```python
from build123d import *

# Parameters (mm, degrees)
SKETCH1_W                     = 965
SKETCH1_H                     = 279
BASE_FLANGE1_DEPTH            = 0.7366
EDGE_FLANGE1_STRIP_W          = 4.4196
EDGE_FLANGE1_STRIP_H          = 0.7366
EDGE_FLANGE1_STRIP_CUT_DEPTH  = 965
EDGE_FLANGE1_DEPTH            = 965
EDGE_FLANGE2_STRIP_W          = 4.4196
EDGE_FLANGE2_STRIP_H          = 0.7366
EDGE_FLANGE2_STRIP_CUT_DEPTH  = 277.5268
EDGE_FLANGE2_DEPTH            = 277.5268
EDGE_FLANGE3_STRIP_W          = 4.4196
EDGE_FLANGE3_STRIP_H          = 0.7366
EDGE_FLANGE3_STRIP_CUT_DEPTH  = 963.5268
EDGE_FLANGE3_DEPTH            = 963.5268
EDGE_FLANGE4_STRIP_W          = 4.4196
EDGE_FLANGE4_STRIP_H          = 0.7366
EDGE_FLANGE4_STRIP_CUT_DEPTH  = 276.0536
EDGE_FLANGE4_DEPTH            = 276.0536
EDGE_FLANGE5_STRIP_W          = 4.4196
EDGE_FLANGE5_STRIP_H          = 0.7366
EDGE_FLANGE5_STRIP_CUT_DEPTH  = 903.1268
EDGE_FLANGE5_RELIEF_W         = 4.7879
EDGE_FLANGE5_RELIEF_H         = 0.3683
EDGE_FLANGE5_RELIEF_CUT_DEPTH = 0.7366
EDGE_FLANGE5_DEPTH            = 903.1268
EDGE_FLANGE6_STRIP_W          = 4.4196
EDGE_FLANGE6_STRIP_H          = 0.7366
EDGE_FLANGE6_STRIP_CUT_DEPTH  = 903.1268
EDGE_FLANGE6_RELIEF_W         = 4.7879
EDGE_FLANGE6_RELIEF_H         = 0.3683
EDGE_FLANGE6_RELIEF_CUT_DEPTH = 0.7366
EDGE_FLANGE6_DEPTH            = 903.1268
EDGE_FLANGE7_STRIP_W          = 4.4196
EDGE_FLANGE7_STRIP_H          = 0.7366
EDGE_FLANGE7_STRIP_CUT_DEPTH  = 276.5902
EDGE_FLANGE7_RELIEF_W         = 4.7879
EDGE_FLANGE7_RELIEF_H         = 0.3683
EDGE_FLANGE7_RELIEF_CUT_DEPTH = 0.7366
EDGE_FLANGE7_DEPTH            = 276.5902
EDGE_FLANGE7_PROFILE_W        = 276.6268
EDGE_FLANGE7_PROFILE_H        = 28.5268
EDGE_FLANGE7_FLAT_DEPTH       = 0.7366
EDGE_FLANGE8_STRIP_W          = 4.4196
EDGE_FLANGE8_STRIP_H          = 0.7366
EDGE_FLANGE8_STRIP_CUT_DEPTH  = 276.0536
EDGE_FLANGE8_DEPTH            = 276.0536


# Sheet-metal steps are written as plain solids
with BuildPart() as part:
    # Sketch1 → Base-Flange1 (new body)
    with BuildSketch(Plane.XY):
        Rectangle(SKETCH1_W, SKETCH1_H)
    extrude(amount=-BASE_FLANGE1_DEPTH)

    # Edge-Flange1 strip (across the edge) → Edge-Flange1 strip cut (cut)
    with BuildSketch(Plane(origin=(-482.5, 139.5, -0.7366), x_dir=(0, -1, 0), z_dir=(1, 0, 0))):
        with Locations((-0.7366, -0.3683)):
            Rectangle(EDGE_FLANGE1_STRIP_W, EDGE_FLANGE1_STRIP_H)
    extrude(amount=EDGE_FLANGE1_STRIP_CUT_DEPTH, mode=Mode.SUBTRACT)

    # Edge-Flange1 section (across the edge) → Edge-Flange1 (add)
    with BuildSketch(Plane(origin=(-482.5, 139.5, -0.7366), x_dir=(0, -1, 0), z_dir=(1, 0, 0))):
        with BuildLine():
            Line((0, 0.7366), (0, 29.2634))
            Line((0, 29.2634), (0.7366, 29.2634))
            Line((0.7366, 29.2634), (0.7366, 0.7366))
            ThreePointArc((0.7366, 0.7366), (0.952345145, 0.215745145), (1.4732, 0))
            Line((1.4732, 0), (1.4732, -0.7366))
            ThreePointArc((1.4732, -0.7366), (0.43149029, -0.30510971), (0, 0.7366))
        make_face()
    extrude(amount=EDGE_FLANGE1_DEPTH)

    # Edge-Flange2 strip (across the edge) → Edge-Flange2 strip cut (cut)
    with BuildSketch(Plane(origin=(482.5, 138.0268, -0.7366), x_dir=(-1, 0, 0), z_dir=(0, -1, 0))):
        with Locations((-0.7366, -0.3683)):
            Rectangle(EDGE_FLANGE2_STRIP_W, EDGE_FLANGE2_STRIP_H)
    extrude(amount=EDGE_FLANGE2_STRIP_CUT_DEPTH, mode=Mode.SUBTRACT)

    # Edge-Flange2 section (across the edge) → Edge-Flange2 (add)
    with BuildSketch(Plane(origin=(482.5, 138.0268, -0.7366), x_dir=(-1, 0, 0), z_dir=(0, -1, 0))):
        with BuildLine():
            Line((0, 0.7366), (0, 29.2634))
            Line((0, 29.2634), (0.7366, 29.2634))
            Line((0.7366, 29.2634), (0.7366, 0.7366))
            ThreePointArc((0.7366, 0.7366), (0.952345145, 0.215745145), (1.4732, 0))
            Line((1.4732, 0), (1.4732, -0.7366))
            ThreePointArc((1.4732, -0.7366), (0.43149029, -0.30510971), (0, 0.7366))
        make_face()
    extrude(amount=EDGE_FLANGE2_DEPTH)

    # Edge-Flange3 strip (across the edge) → Edge-Flange3 strip cut (cut)
    with BuildSketch(Plane(origin=(481.0268, -139.5, -0.7366), x_dir=(0, 1, 0), z_dir=(-1, 0, 0))):
        with Locations((-0.7366, -0.3683)):
            Rectangle(EDGE_FLANGE3_STRIP_W, EDGE_FLANGE3_STRIP_H)
    extrude(amount=EDGE_FLANGE3_STRIP_CUT_DEPTH, mode=Mode.SUBTRACT)

    # Edge-Flange3 section (across the edge) → Edge-Flange3 (add)
    with BuildSketch(Plane(origin=(481.0268, -139.5, -0.7366), x_dir=(0, 1, 0), z_dir=(-1, 0, 0))):
        with BuildLine():
            Line((0, 0.7366), (0, 29.2634))
            Line((0, 29.2634), (0.7366, 29.2634))
            Line((0.7366, 29.2634), (0.7366, 0.7366))
            ThreePointArc((0.7366, 0.7366), (0.952345145, 0.215745145), (1.4732, 0))
            Line((1.4732, 0), (1.4732, -0.7366))
            ThreePointArc((1.4732, -0.7366), (0.43149029, -0.30510971), (0, 0.7366))
        make_face()
    extrude(amount=EDGE_FLANGE3_DEPTH)

    # Edge-Flange4 strip (across the edge) → Edge-Flange4 strip cut (cut)
    with BuildSketch(Plane(origin=(-482.5, -138.0268, -0.7366), x_dir=(1, 0, 0), z_dir=(0, 1, 0))):
        with Locations((-0.7366, -0.3683)):
            Rectangle(EDGE_FLANGE4_STRIP_W, EDGE_FLANGE4_STRIP_H)
    extrude(amount=EDGE_FLANGE4_STRIP_CUT_DEPTH, mode=Mode.SUBTRACT)

    # Edge-Flange4 section (across the edge) → Edge-Flange4 (add)
    with BuildSketch(Plane(origin=(-482.5, -138.0268, -0.7366), x_dir=(1, 0, 0), z_dir=(0, 1, 0))):
        with BuildLine():
            Line((0, 0.7366), (0, 29.2634))
            Line((0, 29.2634), (0.7366, 29.2634))
            Line((0.7366, 29.2634), (0.7366, 0.7366))
            ThreePointArc((0.7366, 0.7366), (0.952345145, 0.215745145), (1.4732, 0))
            Line((1.4732, 0), (1.4732, -0.7366))
            ThreePointArc((1.4732, -0.7366), (0.43149029, -0.30510971), (0, 0.7366))
        make_face()
    extrude(amount=EDGE_FLANGE4_DEPTH)

    # Edge-Flange5 strip (across the edge) → Edge-Flange5 strip cut (cut)
    with BuildSketch(Plane(origin=(451.5634, -138.7634, -30), x_dir=(0, 0, 1), z_dir=(-1, 0, 0))):
        with Locations((-0.7366, -0.3683)):
            Rectangle(EDGE_FLANGE5_STRIP_W, EDGE_FLANGE5_STRIP_H)
    extrude(amount=EDGE_FLANGE5_STRIP_CUT_DEPTH, mode=Mode.SUBTRACT)

    # Edge-Flange5 relief (on the sheet) → Edge-Flange5 relief cut (cut)
    with BuildSketch(Plane(origin=(451.5634, -138.7634, -28.5268), x_dir=(0, 0, 1), z_dir=(0, 1, 0))):
        with Locations((-2.02565, 0.18415)):
            Rectangle(EDGE_FLANGE5_RELIEF_W, EDGE_FLANGE5_RELIEF_H)
        with Locations((-2.02565, -903.31095)):
            Rectangle(EDGE_FLANGE5_RELIEF_W, EDGE_FLANGE5_RELIEF_H)
    extrude(amount=-EDGE_FLANGE5_RELIEF_CUT_DEPTH, mode=Mode.SUBTRACT)

    # Edge-Flange5 section (across the edge) → Edge-Flange5 (add)
    with BuildSketch(Plane(origin=(451.5634, -138.7634, -30), x_dir=(0, 0, 1), z_dir=(-1, 0, 0))):
        with BuildLine():
            Line((0, 0.7366), (0, 29.2634))
            Line((0, 29.2634), (0.7366, 29.2634))
            Line((0.7366, 29.2634), (0.7366, 0.7366))
            ThreePointArc((0.7366, 0.7366), (0.952345145, 0.215745145), (1.4732, 0))
            Line((1.4732, 0), (1.4732, -0.7366))
            ThreePointArc((1.4732, -0.7366), (0.43149029, -0.30510971), (0, 0.7366))
        make_face()
    extrude(amount=EDGE_FLANGE5_DEPTH)

    # Edge-Flange6 strip (across the edge) → Edge-Flange6 strip cut (cut)
    with BuildSketch(Plane(origin=(-451.5634, 138.7634, -30), x_dir=(0, 0, 1), z_dir=(1, 0, 0))):
        with Locations((-0.7366, -0.3683)):
            Rectangle(EDGE_FLANGE6_STRIP_W, EDGE_FLANGE6_STRIP_H)
    extrude(amount=EDGE_FLANGE6_STRIP_CUT_DEPTH, mode=Mode.SUBTRACT)

    # Edge-Flange6 relief (on the sheet) → Edge-Flange6 relief cut (cut)
    with BuildSketch(Plane(origin=(-451.5634, 138.7634, -28.5268), x_dir=(0, 0, 1), z_dir=(0, -1, 0))):
        with Locations((-2.02565, 0.18415)):
            Rectangle(EDGE_FLANGE6_RELIEF_W, EDGE_FLANGE6_RELIEF_H)
        with Locations((-2.02565, -903.31095)):
            Rectangle(EDGE_FLANGE6_RELIEF_W, EDGE_FLANGE6_RELIEF_H)
    extrude(amount=-EDGE_FLANGE6_RELIEF_CUT_DEPTH, mode=Mode.SUBTRACT)

    # Edge-Flange6 section (across the edge) → Edge-Flange6 (add)
    with BuildSketch(Plane(origin=(-451.5634, 138.7634, -30), x_dir=(0, 0, 1), z_dir=(1, 0, 0))):
        with BuildLine():
            Line((0, 0.7366), (0, 29.2634))
            Line((0, 29.2634), (0.7366, 29.2634))
            Line((0.7366, 29.2634), (0.7366, 0.7366))
            ThreePointArc((0.7366, 0.7366), (0.952345145, 0.215745145), (1.4732, 0))
            Line((1.4732, 0), (1.4732, -0.7366))
            ThreePointArc((1.4732, -0.7366), (0.43149029, -0.30510971), (0, 0.7366))
        make_face()
    extrude(amount=EDGE_FLANGE6_DEPTH)

    # Edge-Flange7 strip (across the edge) → Edge-Flange7 strip cut (cut)
    with BuildSketch(Plane(origin=(481.7634, 138.0268, -30), x_dir=(0, 0, 1), z_dir=(0, -1, 0))):
        with Locations((-0.7366, -0.3683)):
            Rectangle(EDGE_FLANGE7_STRIP_W, EDGE_FLANGE7_STRIP_H)
    extrude(amount=EDGE_FLANGE7_STRIP_CUT_DEPTH, mode=Mode.SUBTRACT)

    # Edge-Flange7 relief (on the sheet) → Edge-Flange7 relief cut (cut)
    with BuildSketch(Plane(origin=(481.7634, 138.0268, -28.5268), x_dir=(0, 0, 1), z_dir=(-1, 0, 0))):
        with Locations((-2.02565, -276.77435)):
            Rectangle(EDGE_FLANGE7_RELIEF_W, EDGE_FLANGE7_RELIEF_H)
    extrude(amount=-EDGE_FLANGE7_RELIEF_CUT_DEPTH, mode=Mode.SUBTRACT)

    # Edge-Flange7 bend section (across the edge) → Edge-Flange7 (add)
    with BuildSketch(Plane(origin=(481.7634, 138.0268, -30), x_dir=(0, 0, 1), z_dir=(0, -1, 0))):
        with BuildLine():
            Line((0, 0.7366), (0.7366, 0.7366))
            ThreePointArc((0.7366, 0.7366), (0.952345145, 0.215745145), (1.4732, 0))
            Line((1.4732, 0), (1.4732, -0.7366))
            ThreePointArc((1.4732, -0.7366), (0.43149029, -0.30510971), (0, 0.7366))
        make_face()
    extrude(amount=EDGE_FLANGE7_DEPTH)

    # Edge-Flange7 profile (on flange) → Edge-Flange7 flat (add)
    with BuildSketch(Plane(origin=(481.7634, 0, -30), x_dir=(0, 1, 0), z_dir=(0, 0, 1))):
        with Locations((-0.25, 15)):
            Rectangle(EDGE_FLANGE7_PROFILE_W, EDGE_FLANGE7_PROFILE_H)
    extrude(amount=EDGE_FLANGE7_FLAT_DEPTH)

    # Edge-Flange8 strip (across the edge) → Edge-Flange8 strip cut (cut)
    with BuildSketch(Plane(origin=(-481.7634, -138.0268, -30), x_dir=(0, 0, 1), z_dir=(0, 1, 0))):
        with Locations((-0.7366, -0.3683)):
            Rectangle(EDGE_FLANGE8_STRIP_W, EDGE_FLANGE8_STRIP_H)
    extrude(amount=EDGE_FLANGE8_STRIP_CUT_DEPTH, mode=Mode.SUBTRACT)

    # Edge-Flange8 section (across the edge) → Edge-Flange8 (add)
    with BuildSketch(Plane(origin=(-481.7634, -138.0268, -30), x_dir=(0, 0, 1), z_dir=(0, 1, 0))):
        with BuildLine():
            Line((0, 0.7366), (0, 29.2634))
            Line((0, 29.2634), (0.7366, 29.2634))
            Line((0.7366, 29.2634), (0.7366, 0.7366))
            ThreePointArc((0.7366, 0.7366), (0.952345145, 0.215745145), (1.4732, 0))
            Line((1.4732, 0), (1.4732, -0.7366))
            ThreePointArc((1.4732, -0.7366), (0.43149029, -0.30510971), (0, 0.7366))
        make_face()
    extrude(amount=EDGE_FLANGE8_DEPTH)


solid = part.part
```
Verification items for the finished model (mm, model axes). A direction names the side the tool comes from. Coordinates: 2 decimals unless noted, no trailing zeros. Loops run counter-clockwise (first coordinate to the right, second up) from the corner with the lowest first, then second, coordinate; pieces in that order, holes last. Notation, with made-up numbers: (-30.75, 12.5) - (22.25, 12.5) arc R13 ccw to (22.25, 21.5) - close; hole circle Ø1 at (87, -29.5). An arc over 180 degrees is marked (long way). Return JSON: item names as keys, results as strings.
1. Mould release check, pull along Z, two halves, no side actions. Record for faces 1 (the flat face through (-6, 124, -30)), 2 (the flat face through (6, -138.763, -16)), 3 (the flat face through (6, -139.5, -16)): +Z half, -Z half, draft (parallel to the pull), parting line (faces both ways), or undercut.
Established:
{"face 1": "-Z half", "face 2": "undercut", "face 3": "draft"}
2. Go/stop test with flat-tipped pins: pin 1 (0.6 mm diameter, centred on y = -118.5, z = -29, fed in from -X); pin 2 (0.6 mm diameter, centred on y = -121, z = -29, fed in from +X); pin 3 (23 mm diameter, centred on x = -36.5, y = -121.5, fed in from +Z); pin 4 (4 mm diameter, centred on x = -382, y = 51, fed in from -Z). Record where each tip stops, or that it passes through.
Established:
{"pin 1": "stops at x = -482.49", "pin 2": "stops at x = 482.49", "pin 3": "stops at z = 0", "pin 4": "stops at z = -0.74"}
3. Thickness scan on L1, parallel to X at y = 85.5, z = -10.25; L2, parallel to Y at x = 56.5, z = -21.25; L3, parallel to Z at x = 45, y = -32. Record the ranges inside material, lowest first.
Established:
{"L1": "x = -482.5 to -481.76, 481.76 to 482.5", "L2": "y = -139.5 to -138.76, 138.76 to 139.5", "L3": "z = -0.74 to 0"}
4. Section check A-A, the plane y = 123. Record the boundary of the cut face in (x, z).
Established:
{"outline": "(-482.5, -28.53) arc R1.47 ccw to (-481.03, -30) - (-452.5, -30) - (-452.5, -29.26) - (-481.03, -29.26) arc R0.74 cw to (-481.76, -28.53) - (-481.76, -1.47) arc R0.74 cw to (-481.03, -0.74) - (481.03, -0.74) arc R0.74 cw to (481.76, -1.47) - (481.76, -28.53) arc R0.74 cw to (481.03, -29.26) - (452.5, -29.26) - (452.5, -30) - (481.03, -30) arc R1.47 ccw to (482.5, -28.53) - (482.5, -1.47) arc R1.47 ccw to (481.03, 0) - (-481.03, 0) arc R1.47 ccw to (-482.5, -1.47) - close; (-451.56, -30) - (451.56, -30) - (451.56, -29.26) - (-451.56, -29.26) - close"}
5. Tool access check on faces 4 (the flat face through (467, -2, -30)), 5 (the flat face through (481.763, 1, -16)), 6 (the flat face through (-6, 124, -29.263)). Record the directions out of +Z, -Z, +X, -X, +Y, -Y that give a thin tool (end or side, any length) a straight path to the whole face; none if there is none.
Established:
{"face 4": "-Z, +X, -X, +Y, -Y", "face 5": "-Y", "face 6": "none"}
6. Section check D-D, the plane y = -50. Record the boundary of the cut face in (x, z), then the cut area to 3 significant figures.
Established:
{"outline": "(-482.5, -28.53) arc R1.47 ccw to (-481.03, -30) - (-452.5, -30) - (-452.5, -29.26) - (-481.03, -29.26) arc R0.74 cw to (-481.76, -28.53) - (-481.76, -1.47) arc R0.74 cw to (-481.03, -0.74) - (481.03, -0.74) arc R0.74 cw to (481.76, -1.47) - (481.76, -28.53) arc R0.74 cw to (481.03, -29.26) - (452.5, -29.26) - (452.5, -30) - (481.03, -30) arc R1.47 ccw to (482.5, -28.53) - (482.5, -1.47) arc R1.47 ccw to (481.03, 0) - (-481.03, 0) arc R1.47 ccw to (-482.5, -1.47) - close", "area": "796 mm2"}
7. Section check C-C, the plane x = -388. Record the boundary of the cut face in (y, z).
Established:
{"outline": "(-139.5, -28.53) arc R1.47 ccw to (-138.03, -30) - (-109.5, -30) - (-109.5, -29.26) - (-138.03, -29.26) arc R0.74 cw to (-138.76, -28.53) - (-138.76, -1.47) arc R0.74 cw to (-138.03, -0.74) - (138.03, -0.74) arc R0.74 cw to (138.76, -1.47) - (138.76, -28.53) arc R0.74 cw to (138.03, -29.26) - (109.5, -29.26) - (109.5, -30) - (138.03, -30) arc R1.47 ccw to (139.5, -28.53) - (139.5, -1.47) arc R1.47 ccw to (138.03, 0) - (-138.03, 0) arc R1.47 ccw to (-139.5, -1.47) - close"}
8. Section check B-B, the plane z = -7. Record the boundary of the cut face in (x, y).
Established:
{"outline": "(-482.5, -139.5) - (481.03, -139.5) - (481.03, -138.76) - (-482.5, -138.76) - close; (-482.5, -138.03) - (-481.76, -138.03) - (-481.76, 138.03) - (-482.5, 138.03) - close; (-482.5, 138.76) - (482.5, 138.76) - (482.5, 139.5) - (-482.5, 139.5) - close; (481.76, -139.5) - (482.5, -139.5) - (482.5, 138.03) - (481.76, 138.03) - close"}
